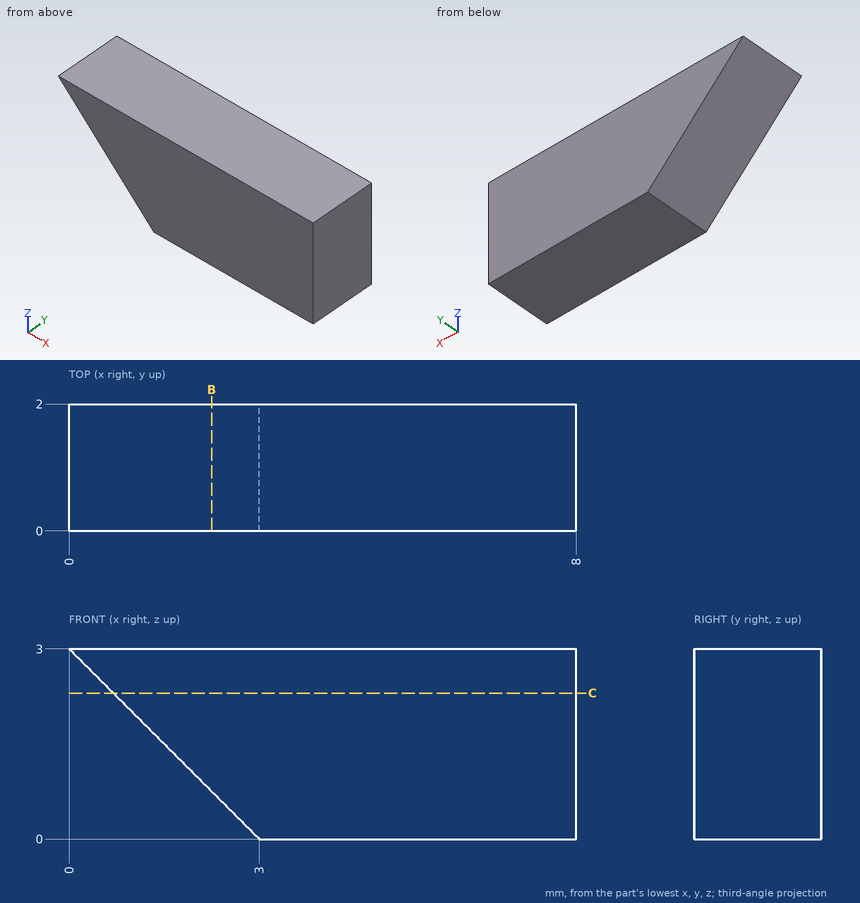
Answer from the drawing. Dimensions are ordinates in mm from the lowest x, y and z of the part. Coordinates: 2 decimals unless noted, no trailing zeros. Order: outer loops, then holes, each group sorted by start corner. A loop starts at its lowest first (then second) coordinate and runs counter-clockwise, first axis right, second up. Notation, with made-up numbers: (-19, -13.75) - (15, -13.75) arc R23 cw to (15, 9.25) - close; hole circle Ø9 at (72.25, 38). An arc over 180 degrees is marked (long way). Answer as a JSON object with one key per item and string values. Group by question number.
Item 1: Consider probe 1 along X at (y, z) = (1.85, 1); probe 2 along X at (y, z) = (0.3, 0.2); probe 3 along Z at (x, y) = (1.75, 1.6). Determine where each line is inside the solid, lowest interval first. Write a range as from..to.
Item 2: Section B-B (x = 2.25) is taken. Give the vertices of the cut face in (y, z).
Item 3: A flat-ended cylindrical pin translates along its axis: P1, Ø1, axis at y = 0.5, z = 1.5, coming from the -X side. Find the tip coordinate at first contact, or state that the pin passes through.
Item 4: Section C-C (z = 2.3) is taken. Give the vertices of the cut face in (x, y), plus the area to 3 significant figures.
Results are:
{
 "1": {"probe 1": "x = 2..8", "probe 2": "x = 2.8..8", "probe 3": "z = 1.25..3"},
 "2": {"outline": "(0, 0.75) - (2, 0.75) - (2, 3) - (0, 3) - close"},
 "3": {"P1": "stops at x = 1"},
 "4": {"outline": "(0.7, 0) - (8, 0) - (8, 2) - (0.7, 2) - close", "area": "14.6 mm^2"}
}
